from build123d import *

# Parameters (mm, degrees)
SKETCH1_W           = 742.95
SKETCH1_H           = 615.95
BOSS_EXTRUDE1_DEPTH = 3.175
SKETCH2_W           = 41.275
SKETCH2_H           = 41.275
SKETCH2_W_2         = 50.8
SKETCH2_H_2         = 50.8
SKETCH2_W_3         = 190.5
SKETCH2_H_3         = 193.675
CUT_EXTRUDE1_DEPTH  = 483.54777678
SKETCH3_W           = 130.175
SKETCH3_H           = 615.95
CUT_EXTRUDE2_DEPTH  = 483.54777678


with BuildPart() as part:
    # Sketch1 → Boss-Extrude1 (new body)
    with BuildSketch(Plane.XY):
        Rectangle(SKETCH1_W, SKETCH1_H)
    extrude(amount=BOSS_EXTRUDE1_DEPTH)

    # Sketch2 → Cut-Extrude1 (cut, through all)
    with BuildSketch(Plane.XY.offset(3.175)):
        with Locations((-350.8375, 287.3375)):
            Rectangle(SKETCH2_W, SKETCH2_H)
        with Locations((-346.075, -282.575)):
            Rectangle(SKETCH2_W_2, SKETCH2_H_2)
        with Locations((220.6625, 287.3375)):
            Rectangle(SKETCH2_W, SKETCH2_H)
        with Locations((146.05, -211.1375)):
            Rectangle(SKETCH2_W_3, SKETCH2_H_3)
    extrude(amount=-CUT_EXTRUDE1_DEPTH, mode=Mode.SUBTRACT)

    # Sketch3 → Cut-Extrude2 (cut, through all)
    with BuildSketch(Plane.XY.offset(3.175)):
        with Locations((306.3875, 0)):
            Rectangle(SKETCH3_W, SKETCH3_H)
    extrude(amount=-CUT_EXTRUDE2_DEPTH, mode=Mode.SUBTRACT)


solid = part.part
Verification items for the finished model (mm, model axes). Coordinates: 2 decimals unless noted, no trailing zeros. Order: outer loops, then holes, each group sorted by start corner. A loop starts at its lowest first (then second) coordinate and runs counter-clockwise, first axis right, second up. Notation, with made-up numbers: M 3.5,40 L 8.5,40 A33 cw 8.5,71 Z; hole C 12,47.25 d11. An arc over 180 degrees is marked long. Return JSON: item names as keys, results as strings.
1) Cross-section at A-A, the plane z = 0.8. Record the boundary of the cut face in (x, y) (3 decimals).
Answer list:
{"outline": "M -371.475,-257.175 L -320.675,-257.175 L -320.675,-307.975 L 50.8,-307.975 L 50.8,-114.3 L 241.3,-114.3 L 241.3,266.7 L 200.025,266.7 L 200.025,307.975 L -330.2,307.975 L -330.2,266.7 L -371.475,266.7 Z"}
2) Thickness scan on L1, parallel to X at y = -183.5, z = 2.05 (3 decimals); L2, parallel to Y at x = 119.5, z = 2.95 (3 decimals); L3, parallel to X at y = -262.5, z = 1.65 (3 decimals). Record the ranges inside material, lowest first. Write a range as [from, to].
Answer list:
{"L1": "[-371.475, 50.8]", "L2": "[-114.3, 307.975]", "L3": "[-320.675, 50.8]"}
3) Cross-section at B-B, the plane x = 86.5. Record the boundary of the cut face in (y, z) (3 decimals).
Answer list:
{"outline": "M -114.3,0 L 307.975,0 L 307.975,3.175 L -114.3,3.175 Z"}
4) Gauge pin test, flat ends, axial feed: pin 1 (1.6 mm diameter, centred on x = 144.5, z = 2, fed in from -Y); pin 2 (1 mm diameter, centred on x = -341, z = 2, fed in from +Y); pin 3 (1 mm diameter, centred on y = -288, z = 1, fed in from -X) (3 decimals). Record the tip position at first contact, or that the pin passes through.
Answer list:
{"pin 1": "y = -114.3", "pin 2": "y = 266.7", "pin 3": "x = -320.675"}
5) Cross-section at C-C, the plane y = -245.5. Record the boundary of the cut face in (x, z) (3 decimals).
Answer list:
{"outline": "M -371.475,0 L 50.8,0 L 50.8,3.175 L -371.475,3.175 Z"}
